Geometry check sheet. Reference: the model listing, model coordinates, mm. A direction names the side the tool comes from. Coordinates: 2 decimals unless noted, no trailing zeros. Write each loop counter-clockwise with the first axis right and the second up, starting at its lowest first coordinate (ties: lowest second). Pieces come first, ordered by that corner, then holes. Notation, with made-up numbers: M 16,-30 L 56,-30 A14 cw 56,-17 Z; hole C -35,-2 d11. An arc over 180 degrees is marked long. Write each question's results on one line, items separated by ' | '.
```python
from build123d import *

# Parameters (mm, degrees)
SKETCH_1_W          = 70
SKETCH_1_H          = 46
EXTRUDE_1_DEPTH     = 4
CUT_EXTRUDE_1_REACH = 44.071
SKETCH_2_R          = 1.6
SKETCH_3_W          = 32
SKETCH_3_H          = 18
EXTRUDE_2_DEPTH     = 5
SKETCH_4_W          = 15
SKETCH_4_H          = 2
EXTRUDE_3_DEPTH     = 10
SKETCH_5_W          = 32
SKETCH_5_H          = 18
EXTRUDE_4_DEPTH     = 3
CUT_EXTRUDE_2_REACH = 77.133
SKETCH_6_R          = 2.03
FILLET_2_R          = 7
CUT_EXTRUDE_3_DEPTH = 5


with BuildPart() as part:
    # 草图1 → 凸台-拉伸1 (new body)
    with BuildSketch(Plane(origin=(0, 0, 0), x_dir=(1, 0, 0), z_dir=(0, 1, 0))):
        Rectangle(SKETCH_1_W, SKETCH_1_H)
    extrude(amount=EXTRUDE_1_DEPTH)

    # 草图2 → 切除-拉伸1 (cut, up to next)
    with BuildSketch(Plane(origin=(0, 4, 0), x_dir=(1, 0, 0), z_dir=(0, 1, 0)), mode=Mode.PRIVATE) as cut_extrude_1_sk1:
        with Locations(Location((-22.5, 13, 0), (0, 0, 270))):
            Circle(SKETCH_2_R)
    cut_extrude_1_tool1 = extrude(cut_extrude_1_sk1.sketch, amount=-CUT_EXTRUDE_1_REACH, mode=Mode.PRIVATE) & part.part
    # 草图2 → 切除-拉伸1 (cut, up to next)
    with BuildSketch(Plane(origin=(0, 4, 0), x_dir=(1, 0, 0), z_dir=(0, 1, 0)), mode=Mode.PRIVATE) as cut_extrude_1_sk2:
        with Locations(Location((22.5, 13, 0), (0, 0, 270))):
            Circle(SKETCH_2_R)
    cut_extrude_1_tool2 = extrude(cut_extrude_1_sk2.sketch, amount=-CUT_EXTRUDE_1_REACH, mode=Mode.PRIVATE) & part.part
    add(cut_extrude_1_tool1.solids().sort_by_distance((-22.5, 4, -13))[0], mode=Mode.SUBTRACT)
    add(cut_extrude_1_tool2.solids().sort_by_distance((22.5, 4, -13))[0], mode=Mode.SUBTRACT)

    # 草图3 → 凸台-拉伸2 (add)
    with BuildSketch(Plane.XY.offset(23)):
        with Locations((0, 9)):
            Rectangle(SKETCH_3_W, SKETCH_3_H)
    extrude(amount=EXTRUDE_2_DEPTH)

    # 草图4 → 凸台-拉伸3 (add)
    with BuildSketch(Plane.XY.offset(28)):
        with Locations((-0.197819001, 1)):
            Rectangle(SKETCH_4_W, SKETCH_4_H)
    extrude(amount=EXTRUDE_3_DEPTH)

    # 草图5 → 凸台-拉伸4 (add)
    with BuildSketch(Plane.XY.offset(38)):
        with Locations((0, 9)):
            Rectangle(SKETCH_5_W, SKETCH_5_H)
    extrude(amount=EXTRUDE_4_DEPTH)

    # 切除-拉伸2: up to this face of the body (flat: up to its plane)
    cut_extrude_2_end = Plane(part.part.faces().sort_by_distance((0, 11, 23))[0])
    # 草图6 → 切除-拉伸2 (cut, up to the picked face)
    with BuildSketch(Plane.XY.offset(41), mode=Mode.PRIVATE) as cut_extrude_2_sk1:
        with Locations((-12, 8)):
            Circle(SKETCH_6_R)
    cut_extrude_2_tool1 = split(extrude(cut_extrude_2_sk1.sketch, amount=-CUT_EXTRUDE_2_REACH, mode=Mode.PRIVATE), bisect_by=cut_extrude_2_end, keep=Keep.BOTH, mode=Mode.PRIVATE)
    # 草图6 → 切除-拉伸2 (cut, up to the picked face)
    with BuildSketch(Plane.XY.offset(41), mode=Mode.PRIVATE) as cut_extrude_2_sk2:
        with Locations((-4, 8)):
            Circle(SKETCH_6_R)
    cut_extrude_2_tool2 = split(extrude(cut_extrude_2_sk2.sketch, amount=-CUT_EXTRUDE_2_REACH, mode=Mode.PRIVATE), bisect_by=cut_extrude_2_end, keep=Keep.BOTH, mode=Mode.PRIVATE)
    # 草图6 → 切除-拉伸2 (cut, up to the picked face)
    with BuildSketch(Plane.XY.offset(41), mode=Mode.PRIVATE) as cut_extrude_2_sk3:
        with Locations((4, 8)):
            Circle(SKETCH_6_R)
    cut_extrude_2_tool3 = split(extrude(cut_extrude_2_sk3.sketch, amount=-CUT_EXTRUDE_2_REACH, mode=Mode.PRIVATE), bisect_by=cut_extrude_2_end, keep=Keep.BOTH, mode=Mode.PRIVATE)
    # 草图6 → 切除-拉伸2 (cut, up to the picked face)
    with BuildSketch(Plane.XY.offset(41), mode=Mode.PRIVATE) as cut_extrude_2_sk4:
        with Locations((12, 8)):
            Circle(SKETCH_6_R)
    cut_extrude_2_tool4 = split(extrude(cut_extrude_2_sk4.sketch, amount=-CUT_EXTRUDE_2_REACH, mode=Mode.PRIVATE), bisect_by=cut_extrude_2_end, keep=Keep.BOTH, mode=Mode.PRIVATE)
    add(cut_extrude_2_tool1.solids().sort_by(Axis((-12, 8, 41), (0, 0, -1)))[0], mode=Mode.SUBTRACT)
    add(cut_extrude_2_tool2.solids().sort_by(Axis((-4, 8, 41), (0, 0, -1)))[0], mode=Mode.SUBTRACT)
    add(cut_extrude_2_tool3.solids().sort_by(Axis((4, 8, 41), (0, 0, -1)))[0], mode=Mode.SUBTRACT)
    add(cut_extrude_2_tool4.solids().sort_by(Axis((12, 8, 41), (0, 0, -1)))[0], mode=Mode.SUBTRACT)

    # 圆角2
    fillet_2_edges = [part.edges().sort_by_distance(p)[0] for p in [
        (-16, 18, 25.5),
        (16, 18, 25.5),
        (-16, 18, 39.5),
        (-16, 0, 39.5),
        (16, 0, 39.5),
        (16, 18, 39.5),
        (35, 2, 23),
        (-35, 2, 23),
        (-35, 2, -23),
        (35, 2, -23),
    ]]
    fillet(fillet_2_edges, radius=FILLET_2_R)

    # 草图10 → 切除-拉伸3 (cut)
    with BuildSketch(Plane.XY.offset(28)):
        with BuildLine():
            Line((-16, 11), (-16, 0))
            Line((-16, 0), (-7.697819001, 0))
            ThreePointArc((-7.697819001, 0), (-13.585443233, 4.189362059), (-16, 11))
        make_face()
        with BuildLine():
            Line((16, 0), (7.697819001, 0))
            ThreePointArc((7.697819001, 0), (13.585443233, 4.189362059), (16, 11))
            Line((16, 11), (16, 0))
        make_face()
    extrude(amount=-CUT_EXTRUDE_3_DEPTH, mode=Mode.SUBTRACT)


solid = part.part
```
Q1. Scan lines: probe 1 along X at (y, z) = (1.3, -13); probe 2 along Y at (x, z) = (4, 24.55); probe 3 along Z at (x, y) = (12, 3.5). Record each from-to range of solid material in increasing order.
Geometry check:
probe 1: x = -35 to -24.1, -20.9 to 20.9, 24.1 to 35 | probe 2: y = 0 to 5.97, 10.03 to 18 | probe 3: z = -23 to 28, 38 to 41
Q2. Access from +Z, -Z, +X, -X, +Y, -Y to the whole of each face (thin tool, end or side, straight path). Record for faces 4 (the flat face through (7.302, 1, 33)), 5 (the flat face through (0, 11, 23)), 6 (the cylindrical face through (-13.523, 4.108, 25.535)).
Geometry check:
face 4: +X, +Y, -Y | face 5: -Z, +X, -X, +Y | face 6: -X, -Y
Q3. Depth check by flat-ended pin: P1, Ø6.5, axis at x = 4, y = 8, coming from the -Z side; P2, Ø3, axis at x = -17.5, y = 2.5, coming from the +Z side; P3, Ø3, axis at x = -4, z = 32, coming from the +Y side. Enter the tip coordinate at first touch or a pass-through.
Geometry check:
P1: stops at z = 23 | P2: stops at z = 23 | P3: stops at y = 2
Q4. Sectioned sample at B-B on x = 4. Record the cut outline in (y, z).
Geometry check:
outline: M 0,-23 L 4,-23 L 4,23 L 5.97,23 L 5.97,28 L 2,28 L 2,38 L 5.97,38 L 5.97,41 L 0,41 Z; M 10.03,23 L 18,23 L 18,28 L 10.03,28 Z; M 10.03,38 L 18,38 L 18,41 L 10.03,41 Z
Q5. Sectioned sample at D-D on y = 13. Record the cut outline in (x, z), and give its area (3 significant figures).
Geometry check:
outline: M -15.71,23 L 15.71,23 L 15.71,28 L -15.71,28 Z; M -15.71,38 L 15.71,38 L 15.71,41 L -15.71,41 Z | area: 251 mm2
Q6. Sectioned sample at C-C on z = -13. Record the cut outline in (x, y), and give its area (3 significant figures).
Geometry check:
outline: M -35,0 L -24.1,0 L -24.1,4 L -35,4 Z; M -20.9,0 L 20.9,0 L 20.9,4 L -20.9,4 Z; M 24.1,0 L 35,0 L 35,4 L 24.1,4 Z | area: 254 mm2
Q7. Sectioned sample at A-A on x = 22.5. Record the cut outline in (y, z).
Geometry check:
outline: M 0,-23 L 4,-23 L 4,-14.6 L 0,-14.6 Z; M 0,-11.4 L 4,-11.4 L 4,23 L 0,23 Z
Q8. Mould release check, pull along Z, two halves, no side actions. Record for faces 1 (the flat face through (-16, 9, 39)), 2 (the flat face through (0, 2, 33)), 3 (the cylindrical face through (32.9, 2, 21)): pulls with the +Z half, pulls with the -Z half, needs draft (parallel to the pull), parting line crosses it, or undercut.
Geometry check:
face 1: needs draft | face 2: undercut | face 3: pulls with the +Z half
